Design review of the part built by this model. Coordinates are the model's own, in mm. Coordinates: 2 decimals unless noted, no trailing zeros. Loops run counter-clockwise (first coordinate to the right, second up) from the corner with the lowest first, then second, coordinate; pieces in that order, holes last. Notation, with made-up numbers: (10.5, 67.25) -> (28.5, 67.25) arc R12 ccw to (28.5, 72.25) -> close; hole circle Ø8 at (13.5, 74.25). An arc over 180 degrees is marked (long way). Use one line per item in the form item = value. Start each with the question number.
1. For pin 1 (4 mm diameter, centred on x = -4.5, y = -5, fed in from +Z); pin 2 (2 mm diameter, centred on x = 0, y = -4.5, fed in from +Z); pin 3 (6.5 mm diameter, centred on y = 0, z = 0, fed in from +X); pin 4 (2 mm diameter, centred on x = -6.5, z = 5.5, fed in from -Y), all flat-tipped, find the tip position at first contact; note any pin that passes through.
2. The part is to be moulded in two halves that separate along Y. For faces 1 (the face through (0.14, -3.905, -0.867)), 2 (the face through (-10.5, -5, 0)), 3 (the face through (0.14, 0.33, -7.493)), say which applies: released by +Y, released by -Y, zero draft, split by the parting line, or undercut.
3. Consider section A-A (z = 0). State the section outline as (x, y) points, then the cut area to 3 significant figures.
4. Consider section B-B (x = 9). State the section outline as (y, z) points.
5. Wall thickness on line 1 (Y direction, x = 2, z = 0); line 2 (Y direction, x = -8, z = 1.5); line 3 (Z direction, x = 5.5, y = -6): over which ranges is each line inside the solid? List them lowest first. Write a range as from..to.
from build123d import *

# Parameters (mm, degrees)
F0_W    = 21
F0_H    = 3.5
F2_SIZE = 0.5


with BuildPart() as f1:
    # F0 (on Front) → F1 (revolve)
    with BuildSketch(Plane.XZ):
        with Locations((0, 5.75)):
            Rectangle(F0_W, F0_H)
    revolve(axis=Axis((-0.426252, 0, 0), (-1, 0, 0)))

    # F2
    f2_edges = [f1.edges().sort_by_distance(p)[0] for p in [
        (10.5, 0, -7.5),
        (10.5, 0, -4),
        (-10.5, 0, -4),
        (-10.5, 0, -7.5),
    ]]
    chamfer(f2_edges, length=F2_SIZE)


solid = f1.part
Geometry check:
q1.pin_1 = 6.87
q1.pin_2 = 6.63
q1.pin_3 = through
q1.pin_4 = -6
q2.face_1 = undercut
q2.face_2 = zero draft
q2.face_3 = split by the parting line
q3.outline = (-10.5, -7) -> (-10, -7.5) -> (10, -7.5) -> (10.5, -7) -> (10.5, -4.5) -> (10, -4) -> (-10, -4) -> (-10.5, -4.5) -> close; (-10.5, 4.5) -> (-10, 4) -> (10, 4) -> (10.5, 4.5) -> (10.5, 7) -> (10, 7.5) -> (-10, 7.5) -> (-10.5, 7) -> close
q3.area = 146 mm²
q4.outline = circle Ø15 at (0, 0); hole circle Ø8 at (0, 0)
q5.line_1 = -7.5..-4, 4..7.5
q5.line_2 = -7.35..-3.71, 3.71..7.35
q5.line_3 = -4.5..4.5
